Autodesk Inventor part; units mm, degrees
ref_plane "YZ Plane" through (0, 0, 0) normal (1, 0, 0) x (0, 1, 0)
ref_plane "XZ Plane" through (0, 0, 0) normal (0, 1, 0) x (-1, 0, 0)
ref_plane "XY Plane" through (0, 0, 0) normal (0, 0, 1) x (1, 0, 0)
sketch "Эскиз1" plane through (0, 0, 0) normal (0, 0, 1) x (1, 0, 0)
  circle A0 centre (0, 0) radius 80
  line L0 (-52.7251, -56.1362) -> (-52.7358, -38.0942) construction
  arc A1 (-51.7364, -37.0936) -> (-52.7358, -38.0942) centre (-51.7358, -38.0936) ccw construction
  line L1 (-51.7364, -37.0936) -> (-13.2571, -37.0709) construction
  arc A2 (-12.2565, -38.0703) -> (-13.2571, -37.0709) centre (-13.2565, -38.0709) ccw construction
  line L2 (-12.2565, -38.0703) -> (-12.2459, -56.1122) construction
  arc A3 (-13.2453, -57.1128) -> (-12.2459, -56.1122) centre (-13.2459, -56.1128) ccw construction
  line L3 (-13.2453, -57.1128) -> (-51.7245, -57.1356) construction
  arc A4 (-52.7251, -56.1362) -> (-51.7245, -57.1356) centre (-51.7251, -56.1356) ccw construction
  circle A5 centre (-11.4805, -27.7164) radius 3.15 construction
  circle A6 centre (-27.7164, 11.4805) radius 3.15 construction
  circle A7 centre (11.4805, 27.7164) radius 3.15 construction
  circle A8 centre (27.7164, -11.4805) radius 3.15 construction
  circle A9 centre (0, 0) radius 12.5
  circle A10 centre (0, 0) radius 39.5 construction
  point P0 (0, 0)
  dimension "d10" = 25
extrude "Выдавливание1" add sketch "Эскиз1" along normal blind 4
sketch "Эскиз2" plane through (0, 0, 0) normal (0, 0, -1) x (-1, 0, 0)
  circle A0 centre (0, 0) radius 80
  line L0 (0, 80) -> (0, -80) construction
  line L1 (2, -75) -> (-2, -75)
  line L2 (-2, -75) -> (-2, 75)
  line L3 (-2, 75) -> (2, 75)
  line L4 (2, 75) -> (2, -75)
  line L5 (2, -75) -> (-2, 75) construction
  line L6 (-2, -75) -> (2, 75) construction
  line L7 (-2, 25) -> (2, 25)
  line L8 (-2, -25) -> (2, -25)
  point P0 (0, -25)
  point P1 (0, 75)
  point P2 (0, 25)
  dimension "d2" = 4
  dimension "d3" = 150
  dimension "d4" = 50
  dimension "d5" = 50
extrude "Выдавливание2" cut sketch "Эскиз2" against normal blind 10 contours L1 L2 L8 L4 | L7 L2 L3 L4
sketch "Эскиз3" plane through (0, 0, 4) normal (0, 0, 1) x (1, 0, 0)
  line L0 (5, 53.408) -> (2, 53.408)
  line L1 (2, 31.408) -> (2, 43.408)
  line L2 (17, 28.408) -> (5, 28.408)
  line L3 (39.1243, 28.408) -> (27, 28.408)
  line L4 (2, 53.408) -> (2, 65.4106)
  line L5 (5, 65.4106) -> (5, 53.408)
  line L6 (2, 65.4106) -> (5, 65.4106)
  line L7 (2, 43.408) -> (5, 43.408)
  line L8 (5, 31.408) -> (2, 31.408)
  line L9 (5, 43.408) -> (5, 31.408)
  line L10 (5, 28.408) -> (5, 31.408)
  line L11 (5, 31.408) -> (17, 31.408)
  line L12 (27, 31.408) -> (38.9975, 31.408)
  line L13 (38.9975, 31.408) -> (39.1243, 28.408)
  line L14 (17, 31.408) -> (17, 28.408)
  line L15 (27, 28.408) -> (27, 31.408)
  line L16 (5, 65.4121) -> (5, 65.4106)
  line L17 (102, 0) -> (-112, 0) construction
  line L18 (5, -53.408) -> (2, -53.408)
  line L19 (2, -31.408) -> (2, -43.408)
  line L20 (17, -28.408) -> (5, -28.408)
  line L21 (39.1243, -28.408) -> (27, -28.408)
  line L22 (2, -53.408) -> (2, -65.4106)
  line L23 (5, -65.4106) -> (5, -53.408)
  line L24 (2, -65.4106) -> (5, -65.4106)
  line L25 (2, -43.408) -> (5, -43.408)
  line L26 (5, -31.408) -> (2, -31.408)
  line L27 (5, -43.408) -> (5, -31.408)
  line L28 (5, -28.408) -> (5, -31.408)
  line L29 (5, -31.408) -> (17, -31.408)
  line L30 (27, -31.408) -> (38.9975, -31.408)
  line L31 (38.9975, -31.408) -> (39.1243, -28.408)
  line L32 (17, -31.408) -> (17, -28.408)
  line L33 (27, -28.408) -> (27, -31.408)
  line L34 (5, -65.4121) -> (5, -65.4106)
  line L35 (0, 116) -> (0, -113) construction
  line L36 (-5, 53.408) -> (-2, 53.408)
  line L37 (-2, 31.408) -> (-2, 43.408)
  line L38 (-17, 28.408) -> (-5, 28.408)
  line L39 (-39.1243, 28.408) -> (-27, 28.408)
  line L40 (-2, 53.408) -> (-2, 65.4106)
  line L41 (-5, 65.4106) -> (-5, 53.408)
  line L42 (-2, 65.4106) -> (-5, 65.4106)
  line L43 (-2, 43.408) -> (-5, 43.408)
  line L44 (-5, 31.408) -> (-2, 31.408)
  line L45 (-5, 43.408) -> (-5, 31.408)
  line L46 (-5, 28.408) -> (-5, 31.408)
  line L47 (-5, 31.408) -> (-17, 31.408)
  line L48 (-27, 31.408) -> (-38.9975, 31.408)
  line L49 (-38.9975, 31.408) -> (-39.1243, 28.408)
  line L50 (-17, 31.408) -> (-17, 28.408)
  line L51 (-27, 28.408) -> (-27, 31.408)
  line L52 (-5, 65.4121) -> (-5, 65.4106)
  line L53 (-17, -31.408) -> (-17, -28.408)
  line L54 (-17, -28.408) -> (-5, -28.408)
  line L55 (-5, -28.408) -> (-5, -31.408)
  line L56 (-5, -31.408) -> (-17, -31.408)
  line L57 (-5, -31.408) -> (-2, -31.408)
  line L58 (-5, -43.408) -> (-5, -31.408)
  line L59 (-2, -31.408) -> (-2, -43.408)
  line L60 (-2, -43.408) -> (-5, -43.408)
  line L61 (-5, -53.408) -> (-2, -53.408)
  line L62 (-5, -65.4106) -> (-5, -53.408)
  line L63 (-5, -65.4121) -> (-5, -65.4106)
  line L64 (-2, -53.408) -> (-2, -65.4106)
  line L65 (-2, -65.4106) -> (-5, -65.4106)
  line L66 (-27, -28.408) -> (-27, -31.408)
  line L67 (-27, -31.408) -> (-38.9975, -31.408)
  line L68 (-38.9975, -31.408) -> (-39.1243, -28.408)
  line L69 (-39.1243, -28.408) -> (-27, -28.408)
  point P0 (0, 0)
extrude "Выдавливание3" cut sketch "Эскиз3" against normal blind 10
properties part number "лицо1"
For this review, take the finished solid that the model builds, in its own axes (mm). Coordinates: 2 decimals unless noted, no trailing zeros. Loops run counter-clockwise (first coordinate to the right, second up) from the corner with the lowest first, then second, coordinate; pieces in that order, holes last. Notation, with made-up numbers: (-34.5, 84) - (23.5, 84) arc R32 ccw to (23.5, 118) - close; hole circle Ø1 at (26.5, 66.25). An arc over 180 degrees is marked (long way). Use a Markdown table: item, result. Add a question column.
Item 1: Mouldability with a two-part tool opening along X and no side actions: class faces 1 (the face through (-17.34, 78.1, 1.97)), 2 (the face through (17, 1, 4)), 3 (the face through (-2, -28, 2)) as pulls with the +X half, pulls with the -X half, needs draft (parallel to the pull), parting line crosses it, or undercut.
Item 2: For line 1 (Y direction, x = 0, z = 2.25); line 2 (Y direction, x = 36, z = 0.2); line 3 (Y direction, x = -27.5, z = 3.55), list the stretches that pass through material, from the lowest coordinate up.
Item 3: Insertion check: pin 1 Ø0.9 at (x, z) = (4, 2) entering from +Y; pin 2 Ø0.9 at (x, z) = (3.5, 2.5) entering from -Y; pin 3 Ø1.2 at (x, z) = (-31, 1) entering from -Y. Each pin has a flat end and moves straight along its axis. Give the tip position at first contact, or say it passes through.
Item 4: We need section C-C (x = 32). Give the boundary of the cut face in (y, z).
Item 5: We need section B-B (y = -45.5). Give the boundary of the cut face in (x, z).
Item 6: We need section A-A (x = 0). Give the boundary of the cut face in (y, z), and give its area (3 significant figures).
Results list:
| question | item | result |
|---|---|---|
| 1 | face 1 | parting line crosses it |
| 1 | face 2 | needs draft |
| 1 | face 3 | undercut |
| 2 | line 1 | y = -80 to -75, -25 to -12.5, 12.5 to 25, 75 to 80 |
| 2 | line 2 | y = -71.44 to -31.41, -28.41 to 28.41, 31.41 to 71.44 |
| 2 | line 3 | y = -75.12 to -31.41, -28.41 to 28.41, 31.41 to 75.12 |
| 3 | pin 1 | stops at y = 79.92 |
| 3 | pin 2 | stops at y = -79.94 |
| 3 | pin 3 | stops at y = -74 |
| 4 | outline | (-73.32, 0) - (-31.41, 0) - (-31.41, 4) - (-73.32, 4) - close; (-28.41, 0) - (28.41, 0) - (28.41, 4) - (-28.41, 4) - close; (31.41, 0) - (73.32, 0) - (73.32, 4) - (31.41, 4) - close |
| 5 | outline | (-65.8, 0) - (-2, 0) - (-2, 4) - (-65.8, 4) - close; (2, 0) - (65.8, 0) - (65.8, 4) - (2, 4) - close |
| 6 | outline | (-80, 0) - (-75, 0) - (-75, 4) - (-80, 4) - close; (-25, 0) - (-12.5, 0) - (-12.5, 4) - (-25, 4) - close; (12.5, 0) - (25, 0) - (25, 4) - (12.5, 4) - close; (75, 0) - (80, 0) - (80, 4) - (75, 4) - close |
| 6 | area | 140 mm^2 |
